Geometry check sheet. Reference: the model listing, model coordinates, mm. Face numbers are marked on the shaded views. A direction names the side the tool comes from. Round coordinates to 2 decimals unless told otherwise and drop trailing zeros. Loops run counter-clockwise (first coordinate to the right, second up) from the corner with the lowest first, then second, coordinate; pieces in that order, holes last. Notation, with made-up numbers: (-24.5, 0.5) - (27.5, 0.5) arc R16 cw to (27.5, 18.5) - close; hole circle Ø1 at (42.25, 12.5). An arc over 180 degrees is marked (long way). Write item = value, one per line.
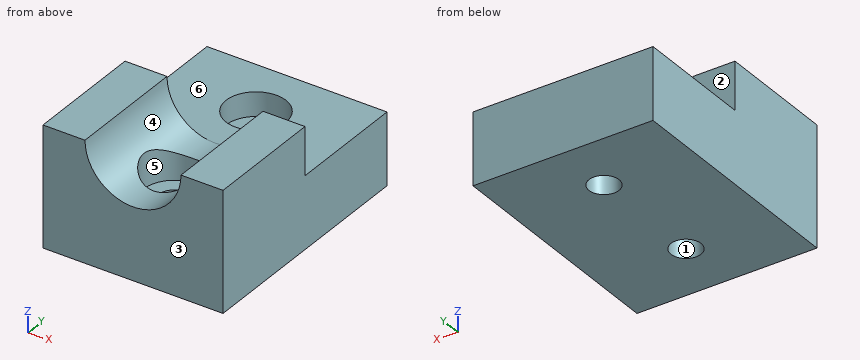
```python
from build123d import *

# Parameters (mm, degrees)
F0_W           = 30
F0_H           = 40
F1_DEPTH       = 20
F7_D           = 5
F7_CBORE_D     = 10
F7_CBORE_DEPTH = 12
F8_DEPTH       = 40
F4_DEPTH       = 20


with BuildPart() as f1:
    # F0 (on Top) → F1 (new body)
    with BuildSketch(Plane.XY):
        Rectangle(F0_W, F0_H)
    extrude(amount=F1_DEPTH)

    # F7 (through all)
    with Locations(Plane.XY.offset(20)):
        with Locations((0, -10), (0, 10)):
            CounterBoreHole(F7_D / 2, F7_CBORE_D / 2, F7_CBORE_DEPTH)

    # F6 (on face) → F8 (cut)
    with BuildSketch(Plane.XZ.offset(20)):
        with BuildLine():
            ThreePointArc((-8, 20), (0, 12), (8, 20))
            Line((8, 20), (-8, 20))
        make_face()
        with BuildLine():
            Line((-8, 20), (8, 20))
            ThreePointArc((8, 20), (0, 28), (-8, 20))
        make_face()
    extrude(amount=-F8_DEPTH, mode=Mode.SUBTRACT)

    # F3 (on face) → F4 (cut)
    with BuildSketch(Plane(origin=(0, 20, 0), x_dir=(-1, 0, 0), z_dir=(0, 1, 0))):
        with BuildLine():
            ThreePointArc((8, 20), (5.6568542495, 14.3431457505), (0, 12))
            Line((0, 12), (15, 12))
            Line((15, 12), (15, 20))
            Line((15, 20), (8, 20))
        make_face()
        with BuildLine():
            Line((-15, 12), (0, 12))
            ThreePointArc((0, 12), (-5.6568542495, 14.3431457505), (-8, 20))
            Line((-8, 20), (-15, 20))
            Line((-15, 20), (-15, 12))
        make_face()
    extrude(amount=-F4_DEPTH, mode=Mode.SUBTRACT)


solid = f1.part
```
(1) Set-up check for the marked faces 4, 5 and 6: record each of +Z, -Z, +X, -X, +Y, -Y from which the full face is reachable in a straight line by a thin tool's end or side.
Answers follow:
face_4 = +Z, +Y, -Y
face_5 = +Z
face_6 = +Z, +X, -X, +Y
(2) Section check C-C (z = 10.5). Enter the section's corners in (x, y).
Answers follow:
outline = (-15, -20) - (15, -20) - (15, 20) - (-15, 20) - close; hole circle Ø10 at (0, -10); hole circle Ø10 at (0, 10)
(3) Gauge pin test, flat ends, axial feed: pin 1 (3 mm diameter, centred on x = 0, y = -10, fed in from -Z); pin 2 (2.5 mm diameter, centred on x = -11, z = 15.5, fed in from +Y); pin 3 (11 mm diameter, centred on x = -1.5, y = 11.5, fed in from +Z); pin 4 (11 mm diameter, centred on x = 1, y = -12, fed in from +Z). Record the tip position at first contact, or that the pin passes through.
Answers follow:
pin_1 = through
pin_2 = 0
pin_3 = 12
pin_4 = 15.34
(4) Section check D-D (y = -2.5). Enter the section's corners in (x, z).
Answers follow:
outline = (-15, 0) - (15, 0) - (15, 20) - (8, 20) arc R8 cw to (-8, 20) - (-15, 20) - close
(5) Section check A-A (y = -10). Enter the section's corners in (x, z) (3 decimals).
Answers follow:
outline = (-15, 0) - (-2.5, 0) - (-2.5, 8) - (-5, 8) - (-5, 13.755) arc R8 cw to (-8, 20) - (-15, 20) - close; (2.5, 0) - (15, 0) - (15, 20) - (8, 20) arc R8 cw to (5, 13.755) - (5, 8) - (2.5, 8) - close
(6) Mould release check, pull along Y, two halves, no side actions. Record for the marked faces 1, 2 and 3: pulls with the +Y half, pulls with the -Y half, needs draft (parallel to the pull), parting line crosses it, or undercut.
Answers follow:
face_1 = undercut
face_2 = pulls with the +Y half
face_3 = pulls with the -Y half
(7) Scan lines: L1, parallel to Y at x = 0, z = 5.75; L2, parallel to Y at x = 0, z = 10.65; L3, parallel to X at y = -10, z = 10.3. Record each from-to range of solid material in increasing order. Write a range as [from, to].
Answers follow:
L1 = [-20, -12.5], [-7.5, 7.5], [12.5, 20]
L2 = [-20, -15], [-5, 5], [15, 20]
L3 = [-15, -5], [5, 15]
(8) Section check B-B (z = 18.25). Enter the section's corners in (x, y), then the cut area to 3 significant figures.
Answers follow:
outline = (-15, -20) - (-7.81, -20) - (-7.81, 0) - (-15, 0) - close; (7.81, -20) - (15, -20) - (15, 0) - (7.81, 0) - close
area = 288 mm²
